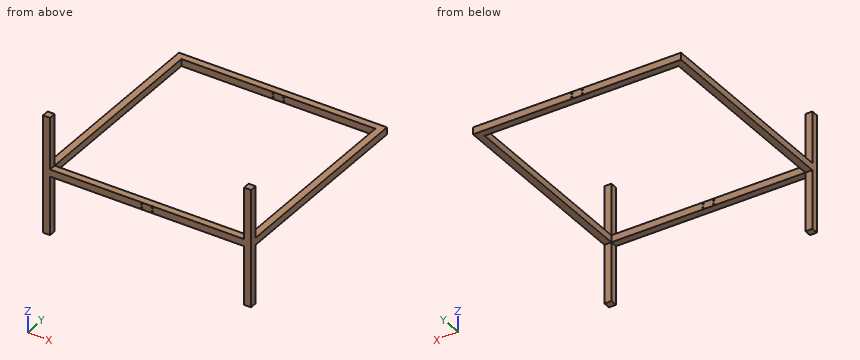
```python
from build123d import *

# Parameters (mm, degrees)
BOSS_EXTRUDE2_DEPTH     = 60
SKETCH2_W               = 60
SKETCH2_H               = 60
BOSS_EXTRUDE3_DEPTH     = 500
SKETCH4_W               = 60
SKETCH4_H               = 60
BOSS_EXTRUDE4_DEPTH     = 1703
CUT_EXTRUDE2_DEPTH      = 1990.302641631
CUT_EXTRUDE2_DEPTH_BACK = 298
SKETCH5_R               = 6


with BuildPart() as part:
    # Sketch1 → Boss-Extrude2 (new body)
    with BuildSketch(Plane.XY):
        Polygon((885, 885), (885, -885), (825, -885), (825, -825), (825, 825), (-825, 825), (-825, -825), (-825, -885), (-885, -885), (-885, 885), align=None)
    extrude(amount=BOSS_EXTRUDE2_DEPTH)

    # Sketch2 → Boss-Extrude3 (add, symmetric)
    with BuildSketch(Plane.XY):
        with Locations((-855, -855)):
            Rectangle(SKETCH2_W, SKETCH2_H)
        with Locations((855, -855)):
            Rectangle(SKETCH2_W, SKETCH2_H)
    extrude(amount=BOSS_EXTRUDE3_DEPTH, both=True)

    # Sketch4 → Boss-Extrude4 (add)
    with BuildSketch(Plane(origin=(-825, 0, 0), x_dir=(0, 0, -1), z_dir=(1, 0, 0))):
        with Locations((-30, -855)):
            Rectangle(SKETCH4_W, SKETCH4_H)
    extrude(amount=BOSS_EXTRUDE4_DEPTH)

    # Sketch5 → Cut-Extrude2 (cut, two sides: drawn at the far end of the back side and taken through both)
    with BuildSketch(Plane.XZ.offset(-825).offset(-CUT_EXTRUDE2_DEPTH_BACK)):
        with Locations(Location((-45, 46, 0), (0, 0, 270))):
            Circle(SKETCH5_R)
        with Locations(Location((-45, 14, 0), (0, 0, 270))):
            Circle(SKETCH5_R)
        with Locations(Location((45, 46, 0), (0, 0, 270))):
            Circle(SKETCH5_R)
        with Locations(Location((45, 14, 0), (0, 0, 270))):
            Circle(SKETCH5_R)
    extrude(amount=CUT_EXTRUDE2_DEPTH + CUT_EXTRUDE2_DEPTH_BACK, mode=Mode.SUBTRACT)


solid = part.part
```
Build history of the part. All positions in model axes, mm. Round coordinates to 2 decimals unless told otherwise and drop trailing zeros. Loops run counter-clockwise (first coordinate to the right, second up) from the corner with the lowest first, then second, coordinate; pieces in that order, holes last. Notation, with made-up numbers: M 7.25,78.25 L 60.25,78.25 A13 ccw 60.25,93.25 Z; hole C 0.25,54 d11. An arc over 180 degrees is marked long. Answer as CSV lines item,"result".
1. Cut at A-A on z = -292.5. Write the cut outline in (x, y).
Resolved:
outline,"M -885,-885 L -825,-885 L -825,-825 L -885,-825 Z; M 825,-885 L 885,-885 L 885,-825 L 825,-825 Z"
2. Cut at B-B on y = 671.5. Write the cut outline in (x, z).
Resolved:
outline,"M -885,0 L -825,0 L -825,60 L -885,60 Z; M 825,0 L 885,0 L 885,60 L 825,60 Z"
3. Flat gauge pins, fed straight in: P1, Ø14, axis at x = 45, z = 14, coming from the -Y side; P2, Ø9.5, axis at x = 45, z = 46, coming from the +Y side. Where does each tip first touch, or does it go through?
Resolved:
P1,"stops at y = -885"
P2,"passes through"
4. Wall check: probe 1 along Z at (x, y) = (-45, 851); probe 2 along X at (y, z) = (-865.5, 46); probe 3 along Y at (x, z) = (-12.5, 30). Give the ranges that are in metal, low to high. Write a range as [from, to].
Resolved:
probe 1,"z = [0, 8], [20, 40], [52, 60]"
probe 2,"x = [-885, -51], [-39, 39], [51, 885]"
probe 3,"y = [-885, -825], [825, 885]"
